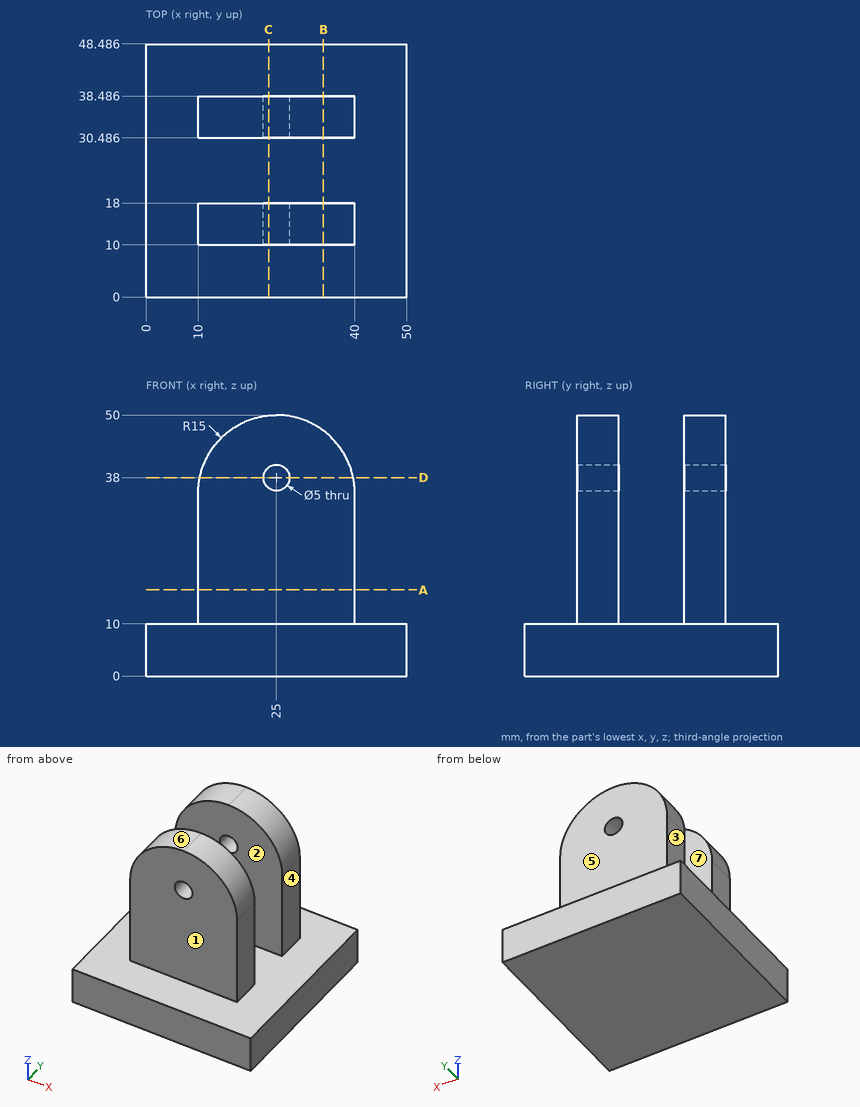
The figure shows three views and two pictorial views of one solid part (mm, origin at its lowest corner). Answer the questions. A direction names the side the tool comes from. Round coordinates to 2 decimals unless told otherwise and drop trailing zeros. Write each loop counter-clockwise with the first axis right and the second up, starting at its lowest first coordinate (ties: lowest second). Pieces come first, ordered by that corner, then holes. Notation, with made-up numbers: (33, 78) -> (68, 78) arc R10 cw to (68, 82) -> close; hole circle Ø7 at (57, 54). An arc over 180 degrees is marked (long way). Answer as a JSON object with one key per item and string values. Group by question number.
Q1. Section A-A (z = 16.5) is taken. Write down the section's boundary in (x, y) (1 decimal).
Q2. Determine the mould class of the marked faces 5, 6 and 7 for opening direction Y: pulls with the +Y half, pulls with the -Y half, needs draft (parallel to the pull), parting line crosses it, or undercut.
Q3. Which of the six approach directions +Z, -Z, +X, -X, +Y, -Y give full straight-line access (tool end or side, diameter ignored) to the marked faces 1, 2, 3 and 4?
Q4. Section D-D (z = 38) is taken. Write down the section's boundary in (x, y) (1 decimal).
Q5. Section C-C (x = 23.5) is taken. Write down the section's boundary in (y, z) (1 decimal).
Q6. Each of these flat-tipped pins is pushed along its axis until it touches: pin 1 Ø2 at (y, z) = (13.5, 43.5) entering from -X; pin 2 Ø9 at (y, z) = (33.5, 22) entering from +X; pin 3 Ø10 at (x, z) = (12, 34) entering from -Y. Where does it stop, or does it pass through?
Q7. Straight lines are drawn through the part: line 1 along Z through (x, y) = (25, 33); line 2 along Y through (x, z) = (32, 24) (1 decimal); line 3 along Z through (x, y) = (8.5, 7). For each, find the intervals that lie inside material, in ascending order.
Q8. Section B-B (x = 34) is taken. Write down the section's boundary in (y, z) (1 decimal).
Check values:
{
 "1": {"outline": "(10, 10) -> (40, 10) -> (40, 18) -> (10, 18) -> close; (10, 30.5) -> (40, 30.5) -> (40, 38.5) -> (10, 38.5) -> close"},
 "2": {"face 5": "pulls with the +Y half", "face 6": "needs draft", "face 7": "undercut"},
 "3": {"face 1": "+Z, +X, -X, -Y", "face 2": "+Z, +X, -X", "face 3": "+Z, -X, +Y, -Y", "face 4": "+Z, +X, +Y, -Y"},
 "4": {"outline": "(10.3, 10) -> (22.5, 10) -> (22.5, 18) -> (10.3, 18) -> close; (10.3, 30.5) -> (22.5, 30.5) -> (22.5, 38.5) -> (10.3, 38.5) -> close; (27.5, 10) -> (39.7, 10) -> (39.7, 18) -> (27.5, 18) -> close; (27.5, 30.5) -> (39.7, 30.5) -> (39.7, 38.5) -> (27.5, 38.5) -> close"},
 "5": {"outline": "(0, 0) -> (48.5, 0) -> (48.5, 10) -> (38.5, 10) -> (38.5, 36) -> (30.5, 36) -> (30.5, 10) -> (18, 10) -> (18, 36) -> (10, 36) -> (10, 10) -> (0, 10) -> close; (10, 40) -> (18, 40) -> (18, 49.9) -> (10, 49.9) -> close; (30.5, 40) -> (38.5, 40) -> (38.5, 49.9) -> (30.5, 49.9) -> close"},
 "6": {"pin 1": "x = 12.01", "pin 2": "x = 40", "pin 3": "y = 10"},
 "7": {"line 1": "0 to 35.5, 40.5 to 50", "line 2": "10 to 18, 30.5 to 38.5", "line 3": "0 to 10"},
 "8": {"outline": "(0, 0) -> (48.5, 0) -> (48.5, 10) -> (38.5, 10) -> (38.5, 47) -> (30.5, 47) -> (30.5, 10) -> (18, 10) -> (18, 47) -> (10, 47) -> (10, 10) -> (0, 10) -> close"}
}
